```python
from build123d import *


with BuildPart() as part:
    # AdditivePipe: sweep along a path in Sketch001
    with BuildLine(Plane.XY) as additivepipe_path:
        Line((14.5, -7.028732), (14, -5.385165))
        ThreePointArc((14, -5.385165), (0, 15), (-14, -5.385165))
        Line((-14, -5.385165), (-14.5, -7.028732))
    # Sketch → AdditivePipe (sweep)
    with BuildSketch(Plane.XZ):
        Polygon((14, 0), (18, 0), (18, 6.5), (14, 6.5), (14, 4.5), (15, 4.5), (15, 2), (14, 2), align=None)
    sweep(path=additivepipe_path.line)


solid = part.part
```
The listing builds one solid part. Answer for the finished solid, in the listing's coordinates (mm). A direction names the side the tool comes from. Give positions to 0.01 mm unless a question says otherwise; leave off trailing zeros. Loops run counter-clockwise (first coordinate to the right, second up) from the corner with the lowest first, then second, coordinate; pieces in that order, holes last. Notation, with made-up numbers: (-9, 65.25) - (23, 65.25) arc R28 ccw to (23, 85.25) - close; hole circle Ø7 at (23.25, 4). An arc over 180 degrees is marked (long way). Return JSON: item names as keys, results as strings. Group by question number.
1. Given pin 1 Ø11 at (x, y) = (-6.5, 9.5) entering from +Z; pin 2 Ø1.5 at (y, z) = (4, 4) entering from -X; pin 3 Ø1 at (y, z) = (-4.5, 3) entering from +X; pin 4 Ø1.5 at (x, z) = (10.5, 5.5) entering from +Y, each flat-ended and moving along its own axis, determine where each tip first touches the part or whether it passes through.
2. Find section C-C (x = 0). Write down the section's boundary in (y, z).
3. Find section B-B (z = 1). Write down the section's boundary in (x, y).
4. Straight lines are drawn through the part: line 1 (X direction, y = 0, z = 1.35); line 2 (X direction, y = 0, z = 3.2); line 3 (Z direction, x = 5.5, y = 13.25). For each, find the intervals that lie inside material, in ascending order. Write a range as [from, to].
5. Which of the six approach directions +Z, -Z, +X, -X, +Y, -Y give full straight-line access (tool end or side, diameter ignored) to faces 5 (the flat face through (-17.053, -7.295, 3.205)), 6 (the flat face through (-14.253, -6.218, 3.268)), 7 (the flat face through (15.46, -7.4, 3.2)), 8 (the flat face through (17.046, -7.272, 3.205))?
6. Find section D-D (y = 14.5). Write down the section's boundary in (x, z), then the cut area to 3 significant figures.
7. Determine the mould class of faces 1 (the flat face through (-1.4, 14.2, 0)), 2 (the flat face through (-13.32, -5.86, 5.51)), 3 (the cylindrical face through (0, 14, 1)), 4 (the flat face through (-1.5, 14.1, 4.5)) for opening direction Y: pulls with the +Y half, pulls with the -Y half, needs draft (parallel to the pull), parting line crosses it, or undercut.
8. Find section A-A (y = 0). Write down the section's boundary in (x, z), then the cut area to 3 significant figures.
Verdict:
{
 "1": {"pin 1": "stops at z = 6.5", "pin 2": "stops at x = -17.7", "pin 3": "stops at x = 17.55", "pin 4": "stops at y = 15.13"},
 "2": {"outline": "(14, 0) - (18, 0) - (18, 6.5) - (14, 6.5) - (14, 4.5) - (15, 4.5) - (15, 2) - (14, 2) - close"},
 "3": {"outline": "(-17.3, -8.11) - (-13.57, -6.67) - (-13.07, -5.03) arc R14 cw (long way) to (13.07, -5.03) - (13.57, -6.67) - (17.3, -8.11) - (16.8, -6.46) arc R18 ccw (long way) to (-16.8, -6.46) - close"},
 "4": {"line 1": "x = [-18, -14], [14, 18]", "line 2": "x = [-18, -15], [15, 18]", "line 3": "z = [0, 2], [4.5, 6.5]"},
 "5": {"face 5": "+Z, -Z, -X", "face 6": "-Y", "face 7": "+Z, -Z, -Y", "face 8": "+Z, -Z, +X"},
 "6": {"outline": "(-10.67, 0) - (10.67, 0) - (10.67, 6.5) - (-10.67, 6.5) - close; hole (-3.84, 2) - (3.84, 2) - (3.84, 4.5) - (-3.84, 4.5) - close", "area": "119 mm^2"},
 "7": {"face 1": "needs draft", "face 2": "pulls with the -Y half", "face 3": "undercut", "face 4": "undercut"},
 "8": {"outline": "(-18, 0) - (-14, 0) - (-14, 2) - (-15, 2) - (-15, 4.5) - (-14, 4.5) - (-14, 6.5) - (-18, 6.5) - close; (14, 0) - (18, 0) - (18, 6.5) - (14, 6.5) - (14, 4.5) - (15, 4.5) - (15, 2) - (14, 2) - close", "area": "47.0 mm^2"}
}
